For this review, use the dimensioned drawing (mm, ordinates from the lowest corner) and the shaded views. Give positions to 0.01 mm unless a question says otherwise; leave off trailing zeros. Order: outer loops, then holes, each group sorted by start corner. A loop starts at its lowest first (then second) coordinate and runs counter-clockwise, first axis right, second up.
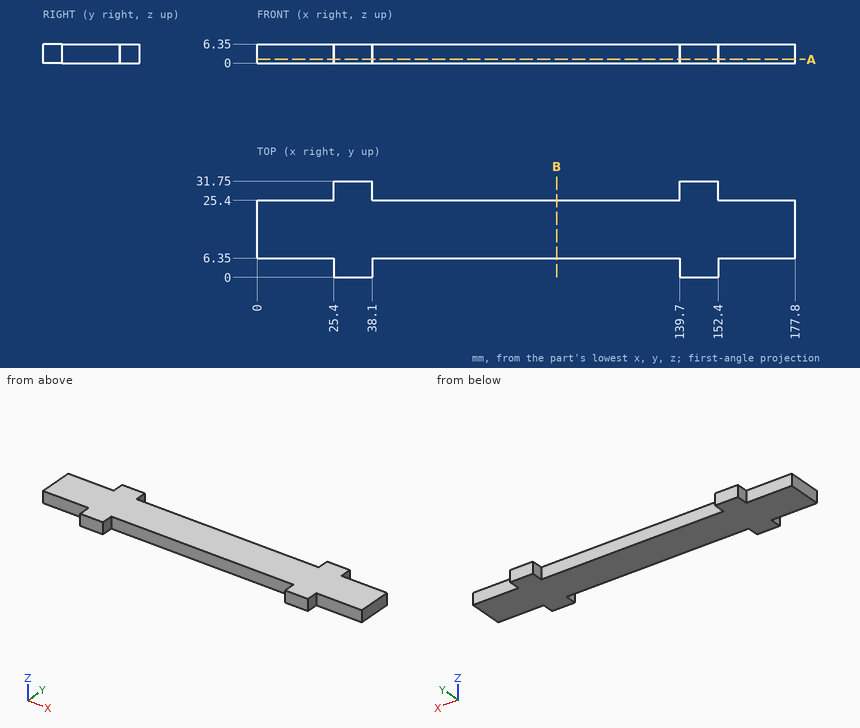
1. Take a section at B-B (x = 99). State the section outline as (y, z) points.
Recorded:
outline: (6.35, 0) - (25.4, 0) - (25.4, 6.35) - (6.35, 6.35) - close
2. For pin 1 (1.9 mm diameter, centred on x = 18.5, z = 4, fed in from -Y); pin 2 (3 mm diameter, centred on x = 138.5, y = 26, fed in from -Z); pin 3 (1.9 mm diameter, centred on y = 30, z = 2, fed in from +X); pin 4 (3 mm diameter, centred on y = 2, z = 2.5, fed in from -X), all flat-tipped, find the tip position at first contact; note any pin that passes through.
Recorded:
pin 1: stops at y = 6.35
pin 2: stops at z = 0
pin 3: stops at x = 152.4
pin 4: stops at x = 25.4
3. For line 1 along X through (y, z) = (4.5, 0.75); line 2 along Y through (x, z) = (11.5, 2.25), list the stretches that pass through material, from the lowest coordinate up.
Recorded:
line 1: x = 25.4 to 38.1, 139.7 to 152.4
line 2: y = 6.35 to 25.4
4. Take a section at A-A (z = 1.25). State the section outline as (x, y) points.
Recorded:
outline: (0, 6.35) - (25.4, 6.35) - (25.4, 0) - (38.1, 0) - (38.1, 6.35) - (139.7, 6.35) - (139.7, 0) - (152.4, 0) - (152.4, 6.35) - (177.8, 6.35) - (177.8, 25.4) - (152.4, 25.4) - (152.4, 31.75) - (139.7, 31.75) - (139.7, 25.4) - (38.1, 25.4) - (38.1, 31.75) - (25.4, 31.75) - (25.4, 25.4) - (0, 25.4) - close
